Verification items for the finished model (mm, model axes). Face numbers are marked on the shaded views. A direction names the side the tool comes from. Give positions to 0.01 mm unless a question says otherwise; leave off trailing zeros. Write each loop counter-clockwise with the first axis right and the second up, starting at its lowest first coordinate (ties: lowest second). Pieces come first, ordered by that corner, then holes.
from build123d import *

# Parameters (mm, degrees)
CORTAR_EXTRUIR1_START = -4
CORTAR_EXTRUIR1_DEPTH = 4
CROQUIS7_W            = 2.599739018
CROQUIS7_H            = 1.208627888
CORTAR_EXTRUIR2_DEPTH = 4


with BuildPart() as part:
    # Croquis1 → Revolución1 (revolve)
    with BuildSketch(Plane(origin=(0, 0, 0), x_dir=(0, 0, -1), z_dir=(1, 0, 0)), mode=Mode.PRIVATE) as revoluci_n1_sk:
        Polygon((0, -4.02), (0, 0), (0, 12.65), (2.423190966, 12.65), (2.423190966, 7.363853001), (1.95, 7.363853001), (1.95, 1.863853001), (3.564484464, 1.863853001), (3.564484464, 0.210352158), (1.95, 0), (1.6, 0), (1.6, -4.02), align=None)
    revolve(revoluci_n1_sk.sketch.rotate(Axis((0, 12.65, 0), (0, -1, 0)), 180), axis=Axis((0, 12.65, 0), (0, -1, 0)))

    # Croquis6 → Cortar-Extruir1 (cut)
    with BuildSketch(Plane(origin=(0, 12.65, 0), x_dir=(1, 0, 0), z_dir=(0, 1, 0)).offset(CORTAR_EXTRUIR1_START)):
        with BuildLine():
            ThreePointArc((2.423190966, 0), (1.985316553, 1.38937851), (0.8299425, 2.276631263))
            Line((0.8299425, 2.276631263), (0.8299425, -2.276631263))
            ThreePointArc((0.8299425, -2.276631263), (1.985316553, -1.38937851), (2.423190966, 0))
        make_face()
        with BuildLine():
            Line((-0.8299425, -2.276631263), (-0.8299425, 2.276631263))
            ThreePointArc((-0.8299425, 2.276631263), (-2.423190966, 0), (-0.8299425, -2.276631263))
        make_face()
    extrude(amount=CORTAR_EXTRUIR1_DEPTH, mode=Mode.SUBTRACT)

    # Croquis7 → Cortar-Extruir2 (cut)
    with BuildSketch(Plane(origin=(0, 12.65, 0), x_dir=(1, 0, 0), z_dir=(0, 1, 0))):
        Rectangle(CROQUIS7_W, CROQUIS7_H)
    extrude(amount=-CORTAR_EXTRUIR2_DEPTH, mode=Mode.SUBTRACT)


solid = part.part
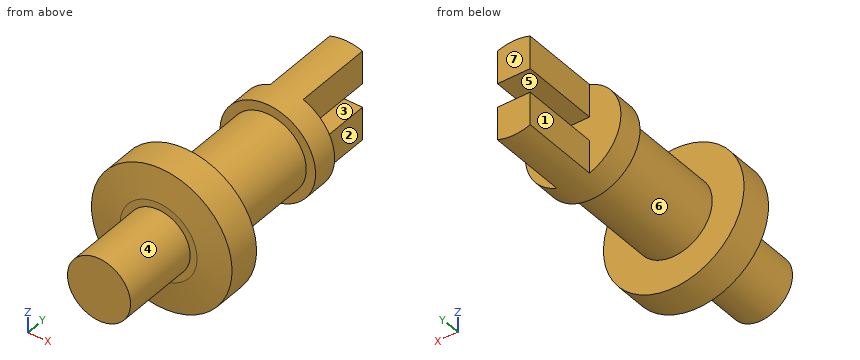
Item 1: Sectioned sample at C-C on x = 0. Record the cut outline in (y, z), then the cut area to 3 significant figures.
Answer key:
outline: (-4.02, -1.6) - (0, -1.6) - (0, -1.95) - (0.21, -3.56) - (1.86, -3.56) - (1.86, -1.95) - (7.36, -1.95) - (7.36, -2.42) - (12.65, -2.42) - (12.65, -0.6) - (8.65, -0.6) - (8.65, 0.6) - (12.65, 0.6) - (12.65, 2.42) - (7.36, 2.42) - (7.36, 1.95) - (1.86, 1.95) - (1.86, 3.56) - (0.21, 3.56) - (0, 1.95) - (0, 1.6) - (-4.02, 1.6) - close
area: 68.0 mm2
Item 2: Sectioned sample at B-B on z = 0. Record the cut outline in (x, y).
Answer key:
outline: (-3.56, 0.21) - (-1.95, 0) - (-1.6, 0) - (-1.6, -4.02) - (1.6, -4.02) - (1.6, 0) - (1.95, 0) - (3.56, 0.21) - (3.56, 1.86) - (1.95, 1.86) - (1.95, 7.36) - (2.42, 7.36) - (2.42, 8.65) - (-2.42, 8.65) - (-2.42, 7.36) - (-1.95, 7.36) - (-1.95, 1.86) - (-3.56, 1.86) - close
Item 3: Scan lines: line 1 along Y through (x, z) = (-2, -1); line 2 along Y through (x, z) = (1.5, -1); line 3 along Y through (x, z) = (1, 0). Record each from-to range of solid material in increasing order.
Answer key:
line 1: y = 0.04 to 1.86, 7.36 to 8.65
line 2: y = 0 to 8.65
line 3: y = -4.02 to 8.65
Item 4: Sectioned sample at A-A on y = 11.25. Record the cut outline in (x, z).
Answer key:
outline: (-0.83, -2.28) arc R2.42 ccw to (0.83, -2.28) - (0.83, -0.6) - (-0.83, -0.6) - close; (-0.83, 0.6) - (0.83, 0.6) - (0.83, 2.28) arc R2.42 ccw to (-0.83, 2.28) - close
Item 5: Sectioned sample at D-D on y = -2. Record the cut outline in (x, z), then the cut area to 3 significant figures.
Answer key:
outline: circle Ø3.2 at (0, 0)
area: 8.04 mm2
Item 6: Release check for a two-part mould opening along Z. For the marked faces 5, 6 and 7 record: released by +Z, released by -Z, zero draft, split by the parting line, or undercut.
Answer key:
face 5: undercut
face 6: split by the parting line
face 7: zero draft
Item 7: Set-up check for the marked faces 1, 2, 3 and 4: record each of +Z, -Z, +X, -X, +Y, -Y from which the full face is reachable in a straight line by a thin tool's end or side.
Answer key:
face 1: +Z, -Z, -X, +Y
face 2: +Z, -Z, +X, +Y
face 3: +X, -X, +Y
face 4: -Y
Item 8: Depth check by flat-ended pin: pin 1 (1.3 mm diameter, centred on y = 10.5, z = 1.5, fed in from -X); pin 2 (1.8 mm diameter, centred on x = 0, y = 10, fed in from +Z); pin 3 (1.3 mm diameter, centred on y = 11, z = -1.5, fed in from +X). Enter the tip coordinate at first touch or a pass-through.
Answer key:
pin 1: stops at x = -0.83
pin 2: stops at z = 2.42
pin 3: stops at x = 0.83
